```python
from build123d import *

# Parameters (mm, degrees)
SZKIC1_R                         = 6
DODANIE_WYCI_GNI_CIE1_DEPTH      = 10
DODANIE_WYCI_GNI_CIE2_DEPTH      = 6
DODANIE_WYCI_GNI_CIE2_DEPTH_BACK = 16
SZKIC2_R                         = 16.5
SZKIC3_R                         = 9
WYTNIJ_WYCI_GNI_CIE1_DEPTH       = 221.098273505
WYTNIJ_WYCI_GNI_CIE2_DEPTH       = 220.579712178
WYTNIJ_WYCI_GNI_CIE2_DEPTH_BACK  = 220.579712178
SZKIC4_R                         = 2.5
ZAOKR_GLENIE1_R                  = 5


with BuildPart() as part:
    # Szkic1 → Dodanie-wyciągnięcie1 (new body)
    with BuildSketch(Plane(origin=(0, 0, 0), x_dir=(1, 0, 0), z_dir=(0, 1, 0))):
        with BuildLine():
            Line((0, 0), (212, 0))
            ThreePointArc((212, 0), (215.535533906, 1.464466094), (217, 5))
            Line((217, 5), (217, 21))
            ThreePointArc((217, 21), (215.535533906, 24.535533906), (212, 26))
            Line((212, 26), (0, 26))
            Line((0, 26), (0, 0))
        make_face()
        with Locations(Location((205, 13, 0), (0, 0, 270))):
            Circle(SZKIC1_R, mode=Mode.SUBTRACT)
    extrude(amount=DODANIE_WYCI_GNI_CIE1_DEPTH)

    # Szkic2 → Dodanie-wyciągnięcie2 (add, two sides: drawn at the far end of the back side and taken through both)
    with BuildSketch(Plane(origin=(0, 10, 0), x_dir=(1, 0, 0), z_dir=(0, 1, 0)).offset(-DODANIE_WYCI_GNI_CIE2_DEPTH_BACK)):
        with Locations(Location((0, 13, 0), (0, 0, 270))):
            Circle(SZKIC2_R)
    extrude(amount=DODANIE_WYCI_GNI_CIE2_DEPTH + DODANIE_WYCI_GNI_CIE2_DEPTH_BACK)

    # Szkic3 → Wytnij-wyciągnięcie1 (cut, through all)
    with BuildSketch(Plane(origin=(0, 16, 0), x_dir=(1, 0, 0), z_dir=(0, 1, 0))):
        with Locations(Location((0, 13, 0), (0, 0, 270))):
            Circle(SZKIC3_R)
    extrude(amount=-WYTNIJ_WYCI_GNI_CIE1_DEPTH, mode=Mode.SUBTRACT)

    # Szkic4 → Wytnij-wyciągnięcie2 (cut, two sides: drawn at the far end of the back side and taken through both)
    with BuildSketch(Plane.XY.offset(-WYTNIJ_WYCI_GNI_CIE2_DEPTH_BACK)):
        with Locations((0, 5)):
            Circle(SZKIC4_R)
    extrude(amount=WYTNIJ_WYCI_GNI_CIE2_DEPTH + WYTNIJ_WYCI_GNI_CIE2_DEPTH_BACK, mode=Mode.SUBTRACT)

    # Zaokrąglenie1
    # the kernel refuses this fillet: 5 mm, written as the material it adds along each edge
    with BuildSketch(Plane(origin=(0, 0, -13), x_dir=(-0.09440175808825453, 0, 0.9955341822709287), z_dir=(-0.9955341822709287, 0, -0.09440175808825453))) as zaokr_glenie1_piece_1_section:
        with BuildLine():
            CenterArc((16.5 + ZAOKR_GLENIE1_R, -ZAOKR_GLENIE1_R), ZAOKR_GLENIE1_R, 90, 90)
            Line((16.5, -ZAOKR_GLENIE1_R), (16.5, 0))
            Line((16.5, 0), (16.5 + ZAOKR_GLENIE1_R, 0))
        make_face()
    zaokr_glenie1_piece_1 = revolve(axis=Axis((0, 0, -13), (0, 1, 0)), revolution_arc=190.833776665, mode=Mode.PRIVATE)
    zaokr_glenie1_piece_1 = split(zaokr_glenie1_piece_1, bisect_by=Plane(origin=(17.924039728, -1.424039728, -26), z_dir=(0, 0, 1)), keep=Keep.TOP, mode=Mode.PRIVATE)
    zaokr_glenie1_piece_1 = split(zaokr_glenie1_piece_1, bisect_by=Plane(origin=(17.924039728, -1.424039728, 0), z_dir=(0, 0, -1)), keep=Keep.TOP, mode=Mode.PRIVATE)
    with BuildSketch(Plane(origin=(0, 10, -13), x_dir=(-0.09440175808827972, 0, 0.9955341822709262), z_dir=(-0.9955341822709262, 0, -0.09440175808827972))) as zaokr_glenie1_piece_2_section:
        with BuildLine():
            CenterArc((16.5 + ZAOKR_GLENIE1_R, ZAOKR_GLENIE1_R), ZAOKR_GLENIE1_R, 180, 90)
            Line((16.5, ZAOKR_GLENIE1_R), (16.5, 0))
            Line((16.5, 0), (16.5 + ZAOKR_GLENIE1_R, 0))
        make_face()
    zaokr_glenie1_piece_2 = revolve(axis=Axis((0, 10, -13), (0, 1, 0)), revolution_arc=190.833776665, mode=Mode.PRIVATE)
    zaokr_glenie1_piece_2 = split(zaokr_glenie1_piece_2, bisect_by=Plane(origin=(17.924039728, 11.424039728, -26), z_dir=(0, 0, 1)), keep=Keep.TOP, mode=Mode.PRIVATE)
    zaokr_glenie1_piece_2 = split(zaokr_glenie1_piece_2, bisect_by=Plane(origin=(17.924039728, 11.424039728, 0), z_dir=(0, 0, -1)), keep=Keep.TOP, mode=Mode.PRIVATE)
    add([zaokr_glenie1_piece_1, zaokr_glenie1_piece_2])


solid = part.part
```
For this review, take the finished solid that the model builds, in its own axes (mm). A direction names the side the tool comes from. Round coordinates to 2 decimals unless told otherwise and drop trailing zeros. Write each loop counter-clockwise with the first axis right and the second up, starting at its lowest first coordinate (ties: lowest second). Pieces come first, ordered by that corner, then holes. Notation, with made-up numbers: (-12, -10) -> (46, -10) arc R10 ccw to (46, -5) -> close; hole circle Ø3 at (50, 46). An arc over 180 degrees is marked (long way). Use one line per item in the form item = value.
Q1. Consider section B-B (y = 5). State the section outline as (x, z) points, then the cut area to 3 significant figures.
Resolved:
outline = (-2.5, -29.31) -> (-2.5, -21.65) arc R9 cw to (-2.5, -4.35) -> (-2.5, 3.31) arc R16.5 ccw to start; (2.5, -29.31) arc R16.5 ccw to (10.16, -26) -> (212, -26) arc R5 ccw to (217, -21) -> (217, -5) arc R5 ccw to (212, 0) -> (10.16, 0) arc R16.5 ccw to (2.5, 3.31) -> (2.5, -4.35) arc R9 cw to (2.5, -21.65) -> close; hole circle Ø12 at (205, -13)
area = 5,660 mm²
Q2. To check wall thickness, follow probe 1 along X at (y, z) = (6, -13); probe 2 along Z at (x, y) = (0, 10.75); probe 3 along Z at (x, y) = (123.5, 4). State the ranges of each line that lie inside material, in increasing order. Write a range as from..to.
Resolved:
probe_1 = -16.5..-9, 9..199, 211..217
probe_2 = -29.5..-22, -4..3.5
probe_3 = -26..0
Q3. Clearance check with flat-ended pins moving along their axes: pin 1 Ø8 at (x, y) = (23, 11) entering from -Z; pin 2 Ø2 at (x, y) = (77, 4.5) entering from +Z; pin 3 Ø10 at (x, z) = (174, -21) entering from -Y; pin 4 Ø4.5 at (x, y) = (0, 5) entering from -Z. State where each tip first meets the part, or that it passes through.
Resolved:
pin_1 = -26
pin_2 = 0
pin_3 = 0
pin_4 = through
Q4. Consider section A-A (z = -13). State the section outline as (x, y) points, then the cut area to 3 significant figures.
Resolved:
outline = (-16.5, -6) -> (-9, -6) -> (-9, 16) -> (-16.5, 16) -> close; (9, -6) -> (16.5, -6) -> (16.5, -5) arc R5 cw to (21.5, 0) -> (199, 0) -> (199, 10) -> (21.5, 10) arc R5 cw to (16.5, 15) -> (16.5, 16) -> (9, 16) -> close; (211, 0) -> (217, 0) -> (217, 10) -> (211, 10) -> close
area = 2,230 mm²
Q5. The part is to be moulded in two halves that separate along X. For faces 4 (the flat face through (-7, 16, -6)), 5 (the cylindrical face through (199.143, 4.93, -14.301)), 6 (the cylindrical face through (-14.64, 4.85, -5.39)), 7 (the cylindrical face through (-0.33, 7.48, -25.63)), say which applies: released by +X, released by -X, zero draft, split by the parting line, or undercut.
Resolved:
face_4 = zero draft
face_5 = undercut
face_6 = split by the parting line
face_7 = undercut
Q6. Machinability: for faces 1 (the flat face through (112, 5, 0)), 2 (the flat face through (110, 5, -26)), 3 (the flat face through (217, 5, -13)), which of the approach directions +Z, -Z, +X, -X, +Y, -Y give a long, thin tool a straight path to every point of the face, cutting with its end or side? Answer none if there is none.
Resolved:
face_1 = +Z, +X, +Y, -Y
face_2 = -Z, +X, +Y, -Y
face_3 = +Z, -Z, +X, +Y, -Y
Q7. Consider section D-D (x = 0). State the section outline as (y, z) points, then the cut area to 3 significant figures.
Resolved:
outline = (-6, -29.5) -> (2.5, -29.5) -> (2.5, -22) -> (-6, -22) -> close; (-6, -4) -> (2.5, -4) -> (2.5, 3.5) -> (-6, 3.5) -> close; (7.5, -29.5) -> (16, -29.5) -> (16, -22) -> (7.5, -22) -> close; (7.5, -4) -> (16, -4) -> (16, 3.5) -> (7.5, 3.5) -> close
area = 255 mm²
Q8. Consider section C-C (x = 205). State the section outline as (y, z) points.
Resolved:
outline = (0, -26) -> (10, -26) -> (10, -19) -> (0, -19) -> close; (0, -7) -> (10, -7) -> (10, 0) -> (0, 0) -> close
